Could you check a few things on this model? Use its own coordinates, in mm. A direction names the side the tool comes from. Coordinates: 2 decimals unless noted, no trailing zeros. Loops run counter-clockwise (first coordinate to the right, second up) from the corner with the lowest first, then second, coordinate; pieces in that order, holes last. Notation, with made-up numbers: (62.5, 22) -> (79.5, 22) arc R19 ccw to (79.5, 43) -> close; hole circle Ø11 at (68, 1). An arc over 180 degrees is marked (long way). One line per question, with ' | ' between items.
Autodesk Inventor part; units mm, degrees
ref_plane "XZ Plane" through (0, 0, 0) normal (0, 1, 0) x (-1, 0, 0)
ref_plane "XY Plane" through (0, 0, 0) normal (0, 0, 1) x (1, 0, 0)
sketch "Sketch1" plane through (0, 0, 0) normal (0, 0, 1) x (1, 0, 0)
  circle A0 centre (0, 0) radius 7.5
  dimension "d0" = 15
extrude "Extrusion1" add sketch "Sketch1" along normal blind 35
hole "Hole1" at (0, 0, 0) direction (0, 0, 1) diameter 6.785 end through all
hole "Hole2" at (0, 0, 35) direction (0, 0, -1) diameter 10 depth 25
chamfer "Chamfer1" distance 0.5 angle 45 1 edges at (-7.5, 0, 35)
ref_plane "Work Plane1" through (7.5, 0, 0) normal (1, 0, 0) x (0, 1, 0)
sketch "Sketch2" plane through (7.5, 0, 0) normal (1, 0, 0) x (0, 1, 0)
  line L0 (-7.5, 0) -> (-7.5, 34.5)
  line L1 (-3.3925, 10) -> (-3.3925, 0)
  line L2 (3.3925, 10) -> (3.3925, 0)
  line L3 (-7.5, 0) -> (7.5, 0)
  line L4 (5, 10) -> (-5, 10)
  line L5 (0, -7) -> (0, 42)
  point P0 (0, 0)
  point P1 (0, 5)
  dimension "d24" = 5
  dimension "d25" = 5
hole "Hole3" at (7.5, 0, 5) direction (-1, 0, 0) diameter 1.694 depth 7.5
properties part number "Screw_Asm_Jig_Upper"
Q1. Please list where these lines run through material, in increasing order: L1, parallel to Y at x = 0, z = 22.75; L2, parallel to Z at x = 0.75, y = -4.25; L3, parallel to Z at x = 5.95, y = 0. Write a range as [from, to].
Values follow:
L1: y = [-7.5, -5], [5, 7.5] | L2: z = [0, 10] | L3: z = [0, 4.15], [5.85, 35]
Q2. We'd pull the mould along Z, two halves only. Please class faces 3 (the face through (-2, 5, 35)), 4 (the face through (5.363, -0.037, 5.846)), 5 (the face through (2, -3, 0)), 6 (the face through (-2.861, 1.824, 5.07)): released by +Z, released by -Z, zero draft, split by the parting line, or undercut.
Values follow:
face 3: released by +Z | face 4: undercut | face 5: released by -Z | face 6: zero draft
Q3. Imagine slicing it at B-B on x = 0. Write out the boundary of the cut face in (y, z), plus the area to 3 significant figures.
Values follow:
outline: (-7.5, 0) -> (-3.39, 0) -> (-3.39, 10) -> (-5, 10) -> (-5, 35) -> (-7, 35) -> (-7.5, 34.5) -> close; (3.39, 0) -> (7.5, 0) -> (7.5, 34.5) -> (7, 35) -> (5, 35) -> (5, 10) -> (3.39, 10) -> close | area: 207 mm2
Q4. Imagine slicing it at C-C on z = 23.5. Write out the boundary of the cut face in (x, y), plus the area to 3 significant figures.
Values follow:
outline: circle Ø15 at (0, 0); hole circle Ø10 at (0, 0) | area: 98.2 mm2
Q5. Imagine slicing it at A-A on y = 0. Write out the boundary of the cut face in (x, z), plus the area to 3 significant figures.
Values follow:
outline: (-7.5, 0) -> (-3.39, 0) -> (-3.39, 10) -> (-5, 10) -> (-5, 35) -> (-7, 35) -> (-7.5, 34.5) -> close; (3.39, 0) -> (7.5, 0) -> (7.5, 4.15) -> (3.39, 4.15) -> close; (3.39, 5.85) -> (7.5, 5.85) -> (7.5, 34.5) -> (7, 35) -> (5, 35) -> (5, 10) -> (3.39, 10) -> close | area: 200 mm2
Q6. For pin 1 (2 mm diameter, centred on x = -4, z = 6.5, fed in from +Y); pin 2 (4 mm diameter, centred on x = -2.5, z = 6.5, fed in from -Y); pin 3 (3 mm diameter, centred on x = -2, z = 24, fed in from +Y), each with a flat end and sliding along its axis, tell me the tip position at first contact or that it passes through.
Values follow:
pin 1: stops at y = 6.87 | pin 2: stops at y = -7.48 | pin 3: stops at y = 7.48
Q7. For faces 1 (the face through (4.88, 1.08, 22.32)), 2 (the face through (-7.493, -0.33, 17.008)), which set-ups out of +Z, -Z, +X, -X, +Y, -Y let a thin tool reach every point of the face, with its end or its side?
Values follow:
face 1: +Z | face 2: +Z, -Z
Q8. Imagine slicing it at D-D on z = 5. Write out the boundary of the cut face in (x, y) (1 decimal).
Values follow:
outline: (3.3, -0.8) arc R3.4 cw (long way) to (3.3, 0.8) -> (7.5, 0.8) arc R7.5 ccw (long way) to (7.5, -0.8) -> close
